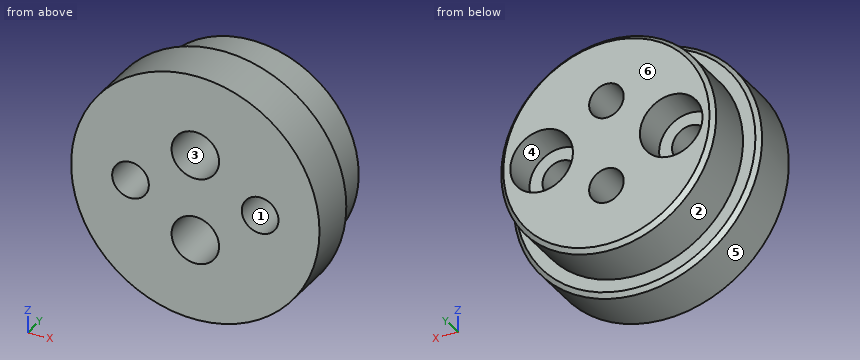
```python
from build123d import *

# Parameters (mm, degrees)
ESQUISSE1_R             = 11.5
ESQUISSE1_R_2           = 1.7
ESQUISSE1_R_3           = 1.6
BOSS_EXTRU_1_DEPTH      = 5
ESQUISSE2_R             = 9.95
ESQUISSE2_R_2           = 1.7
ESQUISSE2_R_3           = 1.6
BOSS_EXTRU_2_DEPTH      = 5
CHANFREIN2_SIZE         = 0.4
CHANFREIN4_SIZE         = 0.4
ESQUISSE3_R             = 2.2
ENL_V_MAT_EXTRU_1_DEPTH = 5.7
ESQUISSE4_R             = 2.9
ENL_V_MAT_EXTRU_2_DEPTH = 3.3


with BuildPart() as part:
    # Esquisse1 → Boss.-Extru.1 (new body)
    with BuildSketch(Plane(origin=(0, 0, 0), x_dir=(1, 0, 0), z_dir=(0, 1, 0))):
        Circle(ESQUISSE1_R)
        with Locations((6, 0)):
            Circle(ESQUISSE1_R_2, mode=Mode.SUBTRACT)
        with Locations((-6, 0)):
            Circle(ESQUISSE1_R_2, mode=Mode.SUBTRACT)
        with Locations((0, 4)):
            Circle(ESQUISSE1_R_3, mode=Mode.SUBTRACT)
        with Locations((0, -4)):
            Circle(ESQUISSE1_R_3, mode=Mode.SUBTRACT)
    extrude(amount=BOSS_EXTRU_1_DEPTH)

    # Esquisse2 → Boss.-Extru.2 (add)
    with BuildSketch(Plane(origin=(0, 5, 0), x_dir=(1, 0, 0), z_dir=(0, 1, 0))):
        Circle(ESQUISSE2_R)
        with Locations((6, 0)):
            Circle(ESQUISSE2_R_2, mode=Mode.SUBTRACT)
        with Locations((-6, 0)):
            Circle(ESQUISSE2_R_2, mode=Mode.SUBTRACT)
        with Locations((0, -4)):
            Circle(ESQUISSE2_R_3, mode=Mode.SUBTRACT)
        with Locations((0, 4)):
            Circle(ESQUISSE2_R_3, mode=Mode.SUBTRACT)
    extrude(amount=BOSS_EXTRU_2_DEPTH)

    # Chanfrein2
    chanfrein2_edges = [part.edges().sort_by_distance(p)[0] for p in [
        (-9.95, 10, 0),
    ]]
    chamfer(chanfrein2_edges, length=CHANFREIN2_SIZE)

    # Chanfrein4
    chanfrein4_edges = [part.edges().sort_by_distance(p)[0] for p in [
        (-11.5, 5, 0),
    ]]
    chamfer(chanfrein4_edges, length=CHANFREIN4_SIZE)

    # Esquisse3 → Enlèv. mat.-Extru.1 (cut)
    with BuildSketch(Plane.XZ):
        with Locations((0, -4)):
            Circle(ESQUISSE3_R)
        with Locations((0, 4)):
            Circle(ESQUISSE3_R)
    extrude(amount=-ENL_V_MAT_EXTRU_1_DEPTH, mode=Mode.SUBTRACT)

    # Esquisse4 → Enlèv. mat.-Extru.2 (cut)
    with BuildSketch(Plane(origin=(0, 10, 0), x_dir=(1, 0, 0), z_dir=(0, 1, 0))):
        with Locations((-6, 0)):
            Circle(ESQUISSE4_R)
        with Locations((6, 0)):
            Circle(ESQUISSE4_R)
    extrude(amount=-ENL_V_MAT_EXTRU_2_DEPTH, mode=Mode.SUBTRACT)


solid = part.part
```
Geometry check sheet. Reference: the model listing, model coordinates, mm. Face numbers are marked on the shaded views. A direction names the side the tool comes from. Coordinates: 2 decimals unless noted, no trailing zeros. Loops run counter-clockwise (first coordinate to the right, second up) from the corner with the lowest first, then second, coordinate; pieces in that order, holes last. Notation, with made-up numbers: (78, -18) - (132, -18) arc R31 cw to (132, 18) - close; hole circle Ø4 at (85.25, 6). An arc over 180 degrees is marked (long way). One line per item, written item: value. Start each with the question number.
(1) Material ranges on line 1 (X direction, y = 8.15, z = 0); line 2 (Z direction, x = 0, y = 8.6); line 3 (Z direction, x = 0, y = 1.75), recorded low to high. Write a range as [from, to].
(2) Cross-section at B-B on y = 9. Enter the section's corners in (x, z).
(3) Tool access check on the marked faces 1, 2 and 3. Record the directions out of +Z, -Z, +X, -X, +Y, -Y that give a thin tool (end or side, any length) a straight path to the whole face; none if there is none.
(4) Mould release check, pull along X, two halves, no side actions. Record for the marked faces 4, 5 and 6: released by +X, released by -X, zero draft, split by the parting line, or undercut.
(5) Cross-section at A-A on x = 0. Enter the section's corners in (y, z).
(6) Depth check by flat-ended pin: P1, Ø4, axis at x = 5, y = 1.5, coming from the -Z side; P2, Ø1.5, axis at y = 2.5, z = -2.5, coming from the +X side; P3, Ø2, axis at x = 4, y = 8, coming from the +Z side. Enter the tip coordinate at first touch or a pass-through.
Results below:
1. line 1: x = [-9.95, -8.9], [-3.1, 3.1], [8.9, 9.95]
1. line 2: z = [-9.95, -5.6], [-2.4, 2.4], [5.6, 9.95]
1. line 3: z = [-11.5, -6.2], [-1.8, 1.8], [6.2, 11.5]
2. outline: circle Ø19.9 at (0, 0); hole circle Ø5.8 at (-6, 0); hole circle Ø3.2 at (0, -4); hole circle Ø3.2 at (0, 4); hole circle Ø5.8 at (6, 0)
3. face 1: +Y, -Y
3. face 2: +Y
3. face 3: -Y
4. face 4: undercut
4. face 5: split by the parting line
4. face 6: zero draft
5. outline: (0, -11.5) - (4.6, -11.5) - (5, -11.1) - (5, -9.95) - (9.6, -9.95) - (10, -9.55) - (10, -5.6) - (5.7, -5.6) - (5.7, -6.2) - (0, -6.2) - close; (0, -1.8) - (5.7, -1.8) - (5.7, -2.4) - (10, -2.4) - (10, 2.4) - (5.7, 2.4) - (5.7, 1.8) - (0, 1.8) - close; (0, 6.2) - (5.7, 6.2) - (5.7, 5.6) - (10, 5.6) - (10, 9.55) - (9.6, 9.95) - (5, 9.95) - (5, 11.1) - (4.6, 11.5) - (0, 11.5) - close
6. P1: stops at z = -11.1
6. P2: stops at x = 11.37
6. P3: stops at z = 9.49
